```python
from build123d import *

# Parameters (mm, degrees)
F0_W         = 5.2
F0_H         = 2
F1_DEPTH     = 2.5
F3_DEPTH     = 2.2
F4_W         = 8
F4_H         = 5
F5_DEPTH     = 2.2
F6_R         = 1.28
F7_DEPTH     = 25
F8_T1_DEPTH  = 1
F8_T3_DEPTH  = 49
F8_T5_DEPTH  = 29.7
F8_T7_DEPTH  = 32.7
F8_S11_W     = 2
F8_S11_H     = 2
F8_T12_DEPTH = 2
F8_S17_W     = 2
F8_S17_H     = 2
F8_T18_DEPTH = 2
F8_S23_W     = 2
F8_S23_H     = 2
F8_T24_DEPTH = 2
F8_S29_W     = 2
F8_S29_H     = 2
F8_T30_DEPTH = 2


# Not quite as in the source:
# - a fillet or chamfer that OpenCascade refuses, or shapes differently, is made with other operations: its cross-section is extruded or revolved along the edge and cut away or added


with BuildPart() as f1:
    # F0 (on Front) → F1 (new body, symmetric)
    with BuildSketch(Plane.XZ):
        Polygon((18.5, 0), (0, 0), (0, -5), (26.5, -5), (26.5, 0), (22.5, 0), align=None)
        Polygon((18.5, 22.5), (18.5, 0), (22.5, 0), (26.5, 0), (26.5, 22.5), (25.1, 22.5), (25.1, 20.5), (19.9, 20.5), (19.9, 22.5), align=None)
        with Locations((22.5, 21.5)):
            Rectangle(F0_W, F0_H)
        Polygon((0, -5), (0, 0), (-18.5, 0), (-22.5, 0), (-26.5, 0), (-26.5, -5), align=None)
        Polygon((-22.5, 0), (-18.5, 0), (-18.5, 22.5), (-19.9, 22.5), (-19.9, 20.5), (-25.1, 20.5), (-25.1, 22.5), (-26.5, 22.5), (-26.5, 0), align=None)
        with Locations((-22.5, 21.5)):
            Rectangle(F0_W, F0_H)
    extrude(amount=F1_DEPTH, both=True)

    # F2 (on face) → F3 (cut)
    with BuildSketch(Plane.XY.offset(22.5)):
        Polygon((19.3823289357, -2.5), (20.8312208665, -2.5), (19.3823289357, -0.011275415), align=None)
        Polygon((20.8312208665, -2.5), (24.1798700484, -2.5), (25.6176710643, 0.011275415), (24.1687791335, 2.5), (20.8201299516, 2.5), (19.3823289357, -0.011275415), align=None)
        Polygon((24.068600328, -2.6943446348), (24.1798700484, -2.5), (20.8312208665, -2.5), (20.9509292637, -2.7056200498), align=None)
        Polygon((24.1798700484, -2.5), (25.6176710643, -2.5), (25.6176710643, 0.011275415), align=None)
        Polygon((-24.1798700484, -2.5), (-20.8312208665, -2.5), (-19.3823289357, -0.011275415), (-20.8201299516, 2.5), (-24.1687791335, 2.5), (-25.6176710643, 0.011275415), align=None)
        Polygon((-20.9509292637, -2.7056200498), (-20.8312208665, -2.5), (-24.1798700484, -2.5), (-24.068600328, -2.6943446348), align=None)
        Polygon((-25.6176710643, -2.5), (-24.1798700484, -2.5), (-25.6176710643, 0.011275415), align=None)
        Polygon((-20.8312208665, -2.5), (-19.3823289357, -2.5), (-19.3823289357, -0.011275415), align=None)
    extrude(amount=-F3_DEPTH, mode=Mode.SUBTRACT)

    # F4 (on face) → F5 (join)
    with BuildSketch(Plane.XY.offset(22.5)):
        with Locations((-22.5, 0)):
            Rectangle(F4_W, F4_H)
        Polygon((25.6176710643, 0.011275415), (24.1687791335, 2.5), (18.5, 2.5), (18.5, -2.5), (25.6176710643, -2.5), align=None)
        Polygon((26.5, -2.5), (26.5, 2.5), (24.1687791335, 2.5), (25.6176710643, 0.011275415), (25.6176710643, -2.5), align=None)
    extrude(amount=F5_DEPTH)

    # F6 (on face) → F7 (cut)
    with BuildSketch(Plane.XY.offset(24.7)):
        with Locations((-22.5, 0)):
            Circle(F6_R)
        with Locations((22.5, 0)):
            Circle(F6_R)
    extrude(amount=-F7_DEPTH, mode=Mode.SUBTRACT)

    # F8: fillet of radius 2 on 12 edges, made by hand

    # F8_s2 → F8_t1 (cut)
    with BuildSketch(Plane.XZ.offset(-0.5)):
        with BuildLine():
            ThreePointArc((-26.5, -3), (-25.9142135624, -4.4142135624), (-24.5, -5))
            Line((-24.5, -5), (-26.5, -5))
            Line((-26.5, -5), (-26.5, -3))
        make_face()
        with BuildLine():
            ThreePointArc((24.5, -5), (25.9142135624, -4.4142135624), (26.5, -3))
            Line((26.5, -3), (26.5, -5))
            Line((26.5, -5), (24.5, -5))
        make_face()
    extrude(amount=F8_T1_DEPTH, mode=Mode.SUBTRACT)

    # F8_s4 → F8_t3 (cut)
    with BuildSketch(Plane.YZ.offset(-24.5)):
        with BuildLine():
            ThreePointArc((2.5, -3), (1.9142135624, -4.4142135624), (0.5, -5))
            Line((0.5, -5), (2.5, -5))
            Line((2.5, -5), (2.5, -3))
        make_face()
        with BuildLine():
            ThreePointArc((-2.5, -3), (-1.9142135624, -4.4142135624), (-0.5, -5))
            Line((-0.5, -5), (-2.5, -5))
            Line((-2.5, -5), (-2.5, -3))
        make_face()
    extrude(amount=F8_T3_DEPTH, mode=Mode.SUBTRACT)

    # F8_s6 → F8_t5 (cut)
    with BuildSketch(Plane.XY):
        with BuildLine():
            ThreePointArc((20.5, -2.5), (19.0857864376, -1.9142135624), (18.5, -0.5))
            Line((18.5, -0.5), (18.5, -2.5))
            Line((18.5, -2.5), (20.5, -2.5))
        make_face()
        with BuildLine():
            ThreePointArc((20.5, 2.5), (19.0857864376, 1.9142135624), (18.5, 0.5))
            Line((18.5, 0.5), (18.5, 2.5))
            Line((18.5, 2.5), (20.5, 2.5))
        make_face()
        with BuildLine():
            ThreePointArc((-18.5, -0.5), (-19.0857864376, -1.9142135624), (-20.5, -2.5))
            Line((-20.5, -2.5), (-18.5, -2.5))
            Line((-18.5, -2.5), (-18.5, -0.5))
        make_face()
        with BuildLine():
            ThreePointArc((-20.5, 2.5), (-19.0857864376, 1.9142135624), (-18.5, 0.5))
            Line((-18.5, 0.5), (-18.5, 2.5))
            Line((-18.5, 2.5), (-20.5, 2.5))
        make_face()
    extrude(amount=F8_T5_DEPTH, mode=Mode.SUBTRACT)

    # F8_s8 → F8_t7 (cut)
    with BuildSketch(Plane.XY.offset(-3)):
        with BuildLine():
            ThreePointArc((24.5, -2.5), (25.9142135624, -1.9142135624), (26.5, -0.5))
            Line((26.5, -0.5), (26.5, -2.5))
            Line((26.5, -2.5), (24.5, -2.5))
        make_face()
        with BuildLine():
            ThreePointArc((24.5, 2.5), (25.9142135624, 1.9142135624), (26.5, 0.5))
            Line((26.5, 0.5), (26.5, 2.5))
            Line((26.5, 2.5), (24.5, 2.5))
        make_face()
        with BuildLine():
            ThreePointArc((-24.5, -2.5), (-25.9142135624, -1.9142135624), (-26.5, -0.5))
            Line((-26.5, -0.5), (-26.5, -2.5))
            Line((-26.5, -2.5), (-24.5, -2.5))
        make_face()
        with BuildLine():
            ThreePointArc((-24.5, 2.5), (-25.9142135624, 1.9142135624), (-26.5, 0.5))
            Line((-26.5, 0.5), (-26.5, 2.5))
            Line((-26.5, 2.5), (-24.5, 2.5))
        make_face()
    extrude(amount=F8_T7_DEPTH, mode=Mode.SUBTRACT)


with BuildPart() as f8_tool10:
    # F8_s11 → F8_t12 (new body)
    with BuildSketch(Plane.XZ.offset(-0.5)):
        with Locations((-25.5, -4)):
            Rectangle(F8_S11_W, F8_S11_H)
    extrude(amount=-F8_T12_DEPTH)

    # F8_s13 → F8_t14 (revolve, cut)
    with BuildSketch(Plane(origin=(-24.5, 0.5, -3), x_dir=(0.7071067812, 0, 0.7071067812), z_dir=(-0.7071067812, 0, 0.7071067812))):
        with BuildLine():
            ThreePointArc((0, -2), (2, 0), (0, 2))
            Line((0, 2), (0, -2))
        make_face()
    revolve(axis=Axis((-24.5, 0.5, -3), (0, 1, 0)), mode=Mode.SUBTRACT)


with BuildPart() as f1_1:
    add(f1.part)

    # F8_t9: cut F8_tool10
    add(f8_tool10.part, mode=Mode.SUBTRACT)


with BuildPart() as f8_tool16:
    # F8_s17 → F8_t18 (new body)
    with BuildSketch(Plane.XZ.offset(0.5)):
        with Locations((-25.5, -4)):
            Rectangle(F8_S17_W, F8_S17_H)
    extrude(amount=F8_T18_DEPTH)

    # F8_s19 → F8_t20 (revolve, cut)
    with BuildSketch(Plane(origin=(-24.5, -0.5, -3), x_dir=(0.7071067812, 0, 0.7071067812), z_dir=(0.7071067812, 0, -0.7071067812))):
        with BuildLine():
            ThreePointArc((0, -2), (2, 0), (0, 2))
            Line((0, 2), (0, -2))
        make_face()
    revolve(axis=Axis((-24.5, -0.5, -3), (0, -1, 0)), mode=Mode.SUBTRACT)


with BuildPart() as f1_2:
    add(f1_1.part)

    # F8_t15: cut F8_tool16
    add(f8_tool16.part, mode=Mode.SUBTRACT)


with BuildPart() as f8_tool22:
    # F8_s23 → F8_t24 (new body)
    with BuildSketch(Plane.YZ.offset(24.5)):
        with Locations((1.5, -4)):
            Rectangle(F8_S23_W, F8_S23_H)
    extrude(amount=F8_T24_DEPTH)

    # F8_s25 → F8_t26 (revolve, cut)
    with BuildSketch(Plane(origin=(24.5, 0.5, -3), x_dir=(0, -0.7071067812, 0.7071067812), z_dir=(0, 0.7071067812, 0.7071067812))):
        with BuildLine():
            ThreePointArc((0, -2), (2, 0), (0, 2))
            Line((0, 2), (0, -2))
        make_face()
    revolve(axis=Axis((24.5, 0.5, -3), (1, 0, 0)), mode=Mode.SUBTRACT)


with BuildPart() as f1_3:
    add(f1_2.part)

    # F8_t21: cut F8_tool22
    add(f8_tool22.part, mode=Mode.SUBTRACT)


with BuildPart() as f8_tool28:
    # F8_s29 → F8_t30 (new body)
    with BuildSketch(Plane.YZ.offset(24.5)):
        with Locations((-1.5, -4)):
            Rectangle(F8_S29_W, F8_S29_H)
    extrude(amount=F8_T30_DEPTH)

    # F8_s31 → F8_t32 (revolve, cut)
    with BuildSketch(Plane(origin=(24.5, -0.5, -3), x_dir=(0, 0.7071067812, 0.7071067812), z_dir=(0, 0.7071067812, -0.7071067812))):
        with BuildLine():
            ThreePointArc((0, -2), (2, 0), (0, 2))
            Line((0, 2), (0, -2))
        make_face()
    revolve(axis=Axis((24.5, -0.5, -3), (1, 0, 0)), mode=Mode.SUBTRACT)


with BuildPart() as f1_4:
    add(f1_3.part)

    # F8_t27: cut F8_tool28
    add(f8_tool28.part, mode=Mode.SUBTRACT)


solid = f1_4.part
```
Design review of the part built by this model. Coordinates are the model's own, in mm. A direction names the side the tool comes from. Give positions to 0.01 mm unless a question says otherwise; leave off trailing zeros. Write each loop counter-clockwise with the first axis right and the second up, starting at its lowest first coordinate (ties: lowest second). Pieces come first, ordered by that corner, then holes. Notation, with made-up numbers: (61.5, 66) - (90.5, 66) arc R21 cw to (90.5, 92) - close; hole circle Ø9 at (65, 26). An arc over 180 degrees is marked (long way). Return JSON: item names as keys, results as strings. Group by question number.
(1) Machinability: for faces 1 (the flat face through (-25.618, -1, 21)), 2 (the cylindrical face through (-0.34, -1.93, -4.4)), 3 (the flat face through (18.5, 0, 13)), 4 (the cylindrical face through (-21.81, 1.08, 10.14)), 5 (the flat face through (-23.44, -1.08, 24.7)), which of the approach directions +Z, -Z, +X, -X, +Y, -Y give a long, thin tool a straight path to every point of the face, cutting with its end or side? Answer none if there is none.
(2) We need section C-C, the plane y = 1.95. Give the boundary of the cut face in (x, z) (1 decimal).
(3) To check wall thickness, follow probe 1 along X at (y, z) = (-0.1, 14.5); probe 2 along Y at (x, z) = (-22.5, 23.85); probe 3 along Z at (x, y) = (-1, 0.2). State the ranges of each line that lie inside material, in increasing order.
(4) Mouldability with a two-part tool opening along X and no side actions: class faces 6 (the flat face through (-23, -2.5, 24)), 7 (the cylindrical face through (23.19, 1.08, 23.62)), 8 (the cylindrical face through (-25.9, 1.93, 10.66)) as +X half, -X half, draft (parallel to the pull), parting line (faces both ways), or undercut.
(5) We need section B-B, the plane x = 22.5. Give the boundary of the cut face in (y, z).
(6) We need section D-D, the plane z = 21.75. Give the boundary of the cut face in (x, y).
(7) We need section A-A, the plane z = 8.75. Give the boundary of the cut face in (x, y).
(8) Insertion check: pin 1 (3 mm diameter, centred on x = -22.5, y = 0, fed in from +Z); pin 2 (1.5 mm diameter, centred on x = 18, z = 9, fed in from -Y); pin 3 (1.3 mm diameter, centred on x = -22.5, y = 0, fed in from +Z). Each pin has a flat end and moves straight along its axis. Give the tip position at first contact, or say it passes through.
Reported:
{
 "1": {"face 1": "-Y", "face 2": "-Z, +X, -X, -Y", "face 3": "+Z, +Y, -Y", "face 4": "+Z", "face 5": "+Z, +X, -X, +Y, -Y"},
 "2": {"outline": "(-25.9, -3) arc R1.4 ccw to (-24.5, -4.4) - (24.5, -4.4) arc R1.4 ccw to (25.9, -3) - (25.9, 24.7) - (19.1, 24.7) - (19.1, 0) - (-19.1, 0) - (-19.1, 24.7) - (-25.9, 24.7) - close; hole (-24.5, 20.3) - (-20.5, 20.3) - (-20.5, 22.5) - (-24.5, 22.5) - close; hole (20.5, 20.3) - (24.5, 20.3) - (24.5, 22.5) - (20.5, 22.5) - close"},
 "3": {"probe 1": "x = -26.5 to -23.78, -21.22 to -18.5, 18.5 to 21.22, 23.78 to 26.5", "probe 2": "y = -2.5 to -1.28, 1.28 to 2.5", "probe 3": "z = -5 to 0"},
 "4": {"face 6": "draft", "face 7": "undercut", "face 8": "-X half"},
 "5": {"outline": "(-2.5, -3) arc R2 ccw to (-0.5, -5) - (0.5, -5) arc R2 ccw to (2.5, -3) - (2.5, 20.3) - (1.28, 20.3) - (1.28, -0.3) - (-1.28, -0.3) - (-1.28, 20.3) - (-2.5, 20.3) - close; (-2.5, 22.5) - (-1.28, 22.5) - (-1.28, 24.7) - (-2.5, 24.7) - close; (1.28, 22.5) - (2.5, 22.5) - (2.5, 24.7) - (1.28, 24.7) - close"},
 "6": {"outline": "(-26.5, -0.5) arc R2 ccw to (-25.62, -2.16) - (-25.62, 0.01) - (-24.17, 2.5) - (-24.5, 2.5) arc R2 ccw to (-26.5, 0.5) - close; (-20.82, 2.5) - (-19.38, -0.01) - (-19.38, -2.16) arc R2 ccw to (-18.5, -0.5) - (-18.5, 0.5) arc R2 ccw to (-20.5, 2.5) - close; (18.5, -0.5) arc R2 ccw to (19.38, -2.16) - (19.38, -0.01) - (20.82, 2.5) - (20.5, 2.5) arc R2 ccw to (18.5, 0.5) - close; (24.17, 2.5) - (25.62, 0.01) - (25.62, -2.16) arc R2 ccw to (26.5, -0.5) - (26.5, 0.5) arc R2 ccw to (24.5, 2.5) - close"},
 "7": {"outline": "(-26.5, -0.5) arc R2 ccw to (-24.5, -2.5) - (-20.5, -2.5) arc R2 ccw to (-18.5, -0.5) - (-18.5, 0.5) arc R2 ccw to (-20.5, 2.5) - (-24.5, 2.5) arc R2 ccw to (-26.5, 0.5) - close; (18.5, -0.5) arc R2 ccw to (20.5, -2.5) - (24.5, -2.5) arc R2 ccw to (26.5, -0.5) - (26.5, 0.5) arc R2 ccw to (24.5, 2.5) - (20.5, 2.5) arc R2 ccw to (18.5, 0.5) - close; hole circle Ø2.56 at (-22.5, 0); hole circle Ø2.56 at (22.5, 0)"},
 "8": {"pin 1": "stops at z = 24.7", "pin 2": "stops at y = -1.47", "pin 3": "stops at z = -0.3"}
}
